```python
from build123d import *

# Parameters (mm, degrees)
F0_W     = 254
F0_H     = 50.8
F1_DEPTH = 152.4
F2_DEPTH = 19.05
F0_R     = 44.45
F3_DEPTH = 127
F5_DEPTH = 9.525


with BuildPart() as f1:
    # F0 (on Front) → F1 (new body)
    with BuildSketch(Plane.XZ):
        with Locations((0, -129.828695)):
            Rectangle(F0_W, F0_H)
    extrude(amount=F1_DEPTH)

    # F0 (on Front) → F2 (join)
    with BuildSketch(Plane.XZ):
        with Locations((0, -129.828695)):
            Rectangle(F0_W, F0_H)
        with BuildLine():
            Line((-59.227747, 70.869428), (-127, -104.428695))
            Line((-127, -104.428695), (127, -104.428695))
            Line((127, -104.428695), (59.227747, 70.869428))
            ThreePointArc((59.227747, 70.869428), (62.4228, 59.617937), (63.5, 47.971305))
            ThreePointArc((63.5, 47.971305), (-11.646632, -14.451495), (-59.227747, 70.869428))
        make_face()
    extrude(amount=F2_DEPTH)

    # F0 (on Front) → F3 (join)
    with BuildSketch(Plane.XZ):
        with BuildLine():
            ThreePointArc((59.227747, 70.869428), (0, 111.471305), (-59.227747, 70.869428))
            ThreePointArc((-59.227747, 70.869428), (-11.646632, -14.451495), (63.5, 47.971305))
            ThreePointArc((63.5, 47.971305), (62.4228, 59.617937), (59.227747, 70.869428))
        make_face()
        with Locations((0, 47.971305)):
            Circle(F0_R, mode=Mode.SUBTRACT)
    extrude(amount=F3_DEPTH)

    # F4 (on Right) → F5 (join, symmetric)
    with BuildSketch(Plane.YZ):
        Polygon((-13.847807, -10.107701), (-107.95, -11.26233), (-107.95, -113.015743), (-13.847807, -113.015743), align=None)
    extrude(amount=F5_DEPTH, both=True)


solid = f1.part
```
The listing builds one solid part. Answer for the finished solid, in the listing's coordinates (mm). A direction names the side the tool comes from. Give positions to 0.01 mm unless a question says otherwise; leave off trailing zeros. Write each loop counter-clockwise with the first axis right and the second up, starting at its lowest first coordinate (ties: lowest second). Pieces come first, ordered by that corner, then holes. Notation, with made-up numbers: (4, -1) - (41, -1) arc R16 cw to (41, 10) - close; hole circle Ø9 at (2.5, 78). An arc over 180 degrees is marked (long way). Use one line per item in the form item = value. Start each with the question number.
1) Find section D-D on z = 79. Determine the outline of the cut face in (x, y).
2) The mould has two halves that part along Z. Classify faces 1 (the face through (-56, -19.05, -55)), 2 (the face through (-92.64, -9.39, -15.55)), 3 (the face through (-127, -75, -130)): pulls with the +Z half, pulls with the -Z half, needs draft (parallel to the pull), parting line crosses it, or undercut.
3) A tool of negligible diameter and unlimited length cuts with its end or side. For faces 4 (the face through (-9.525, -64, -59)), 5 (the face through (62.453, -72.269, 59.457)), 6 (the face through (0, -107.95, -59)), from which of +Z, -Z, +X, -X, +Y, -Y can it reach the whole face along a straight path? Write none if from no direction.
4) Flat-ended cylindrical pins translate along their axes: pin 1 Ø5.5 at (x, z) = (-3, -63) entering from -Y; pin 2 Ø4 at (x, y) = (-85, -26) entering from +Z; pin 3 Ø8 at (x, z) = (-87, -44) entering from +Y; pin 4 Ø5 at (x, z) = (55.5, -2) entering from -Y. Find the tip coordinate at first contact, or state that the pin passes through.
5) Find section C-C on y = -12.5. Determine the outline of the cut face in (x, z).
6) Consider line 1 along Z through (x, y) = (0, -27); line 2 along X through (y, z) = (-62.5, 49); line 3 along Z through (x, y) = (-76, -30.5). Determine where each line is inside the solid, lowest interval first. Write a range as from..to.
7) Find section B-B on y = -111.5. Determine the outline of the cut face in (x, z).
8) Find section A-A on x = 0. Determine the outline of the cut face in (y, z), plus the area to 3 significant figures.
Geometry results:
q1.outline = (-55.4, -127) - (-31.83, -127) - (-31.83, 0) - (-55.4, 0) - close; (31.83, -127) - (55.4, -127) - (55.4, 0) - (31.83, 0) - close
q2.face_1 = undercut
q2.face_2 = pulls with the +Z half
q2.face_3 = needs draft
q3.face_4 = -X, -Y
q3.face_5 = +Z, +X, -Y
q3.face_6 = +X, -X, -Y
q4.pin_1 = -107.95
q4.pin_2 = -104.43
q4.pin_3 = 0
q4.pin_4 = -19.05
q5.outline = (-127, -155.23) - (127, -155.23) - (127, -104.43) - (59.23, 70.87) arc R63.5 ccw to (-59.23, 70.87) - (-127, -104.43) - close; hole circle Ø88.9 at (0, 47.97)
q6.line_1 = -155.23..3.52, 92.42..111.47
q6.line_2 = -63.49..-44.44, 44.44..63.49
q6.line_3 = -155.23..-104.43
q7.outline = (-127, -155.23) - (127, -155.23) - (127, -104.43) - (-127, -104.43) - close; (59.23, 70.87) arc R63.5 ccw (long way) to (63.5, 47.97) arc R63.5 ccw to start; hole circle Ø88.9 at (0, 47.97)
q8.outline = (-152.4, -155.23) - (0, -155.23) - (0, 3.52) - (-127, 3.52) - (-127, -15.53) - (-107.95, -15.53) - (-107.95, -104.43) - (-152.4, -104.43) - close; (-127, 92.42) - (0, 92.42) - (0, 111.47) - (-127, 111.47) - close
q8.area = 22,200 mm2
